The model under review builds one solid part; all positions refer to its coordinate system, in mm. Coordinates: 2 decimals unless noted, no trailing zeros. Order: outer loops, then holes, each group sorted by start corner. A loop starts at its lowest first (then second) coordinate and runs counter-clockwise, first axis right, second up. Notation, with made-up numbers: M 50.25,-11.75 L 57.25,-11.75 A12 ccw 57.25,2.25 Z; hole C 71.5,-5 d6. An arc over 180 degrees is marked long. Answer as CSV lines item,"result". Start each with the question number.
Q1. Wall thickness on L1, parallel to X at y = 230, z = -3; L2, parallel to X at y = 142.5, z = -1.6; L3, parallel to X at y = 96, z = -0.85: over which ranges is each line inside the solid? List them lowest first. Write a range as [from, to].
Q2. Consider section A-A on x = 41. Write out the cut boundary in (y, z), and give its area (3 significant figures).
Q3. Consider section B-B on y = 212.5. Write out the cut boundary in (x, z).
Autodesk Inventor part; units mm, degrees
ref_plane "YZ Plane" through (0, 0, 0) normal (1, 0, 0) x (0, 1, 0)
ref_plane "XZ Plane" through (0, 0, 0) normal (0, 1, 0) x (-1, 0, 0)
ref_plane "XY Plane" through (0, 0, 0) normal (0, 0, 1) x (1, 0, 0)
sketch "Sketch1" plane through (0, 0, 0) normal (0, 0, 1) x (1, 0, 0)
  line L0 (120, -66) -> (20, -66) construction
  line L1 (20, -66) -> (20, -26) construction
  line L2 (20, -26) -> (120, -26) construction
  line L3 (120, -26) -> (120, -66) construction
  line L4 (-275, -71) -> (125, -71) construction
  line L5 (125, -71) -> (125, 329) construction
  line L6 (125, 329) -> (-275, 329) construction
  line L7 (-275, 329) -> (-275, -71) construction
  line L8 (50, 104) -> (50, 154) construction
  line L9 (50, 154) -> (54, 154) construction
  line L10 (54, 154) -> (54, 104) construction
  line L11 (54, 104) -> (50, 104) construction
  line L12 (-50, 254) -> (-100, 254) construction
  line L13 (-100, 254) -> (-100, 258) construction
  line L14 (-100, 258) -> (-50, 258) construction
  line L15 (-50, 258) -> (-50, 254) construction
  line L16 (50, 258) -> (50, 254) construction
  line L17 (50, 254) -> (54, 254) construction
  line L18 (54, 254) -> (54, 204) construction
  line L19 (54, 204) -> (50, 204) construction
  line L20 (50, 204) -> (50, 254) construction
  line L21 (50, 254) -> (0, 254) construction
  line L22 (0, 254) -> (0, 258) construction
  line L23 (0, 258) -> (50, 258) construction
  line L24 (54, 4) -> (50, 4) construction
  line L25 (50, 4) -> (50, 0) construction
  line L26 (50, 0) -> (0, 0) construction
  line L27 (0, 0) -> (0, 4) construction
  line L28 (0, 4) -> (50, 4) construction
  line L29 (50, 4) -> (50, 54) construction
  line L30 (50, 54) -> (54, 54) construction
  line L31 (54, 54) -> (54, 4) construction
  line L32 (-100, 4) -> (-50, 4) construction
  line L33 (-50, 4) -> (-50, 0) construction
  line L34 (-50, 0) -> (-100, 0) construction
  line L35 (-100, 0) -> (-100, 4) construction
  line L36 (-204, 254) -> (-200, 254) construction
  line L37 (-200, 254) -> (-200, 258) construction
  line L38 (-200, 258) -> (-150, 258) construction
  line L39 (-150, 258) -> (-150, 254) construction
  line L40 (-150, 254) -> (-200, 254) construction
  line L41 (-200, 254) -> (-200, 204) construction
  line L42 (-200, 204) -> (-204, 204) construction
  line L43 (-204, 204) -> (-204, 254) construction
  line L44 (-200, 154) -> (-200, 104) construction
  line L45 (-200, 104) -> (-204, 104) construction
  line L46 (-204, 104) -> (-204, 154) construction
  line L47 (-204, 154) -> (-200, 154) construction
  line L48 (-200, 54) -> (-200, 4) construction
  line L49 (-200, 4) -> (-150, 4) construction
  line L50 (-150, 4) -> (-150, 0) construction
  line L51 (-150, 0) -> (-200, 0) construction
  line L52 (-200, 0) -> (-200, 4) construction
  line L53 (-200, 4) -> (-204, 4) construction
  line L54 (-204, 4) -> (-204, 54) construction
  line L55 (-204, 54) -> (-200, 54) construction
  line L56 (-275, -71) -> (125, -71) construction
  line L57 (125, -71) -> (125, 329) construction
  line L58 (125, 329) -> (-275, 329) construction
  line L59 (-275, 329) -> (-275, -71) construction
  line L60 (-275, -71) -> (125, 329) construction
  line L61 (75, 279) -> (-225, 279)
  line L62 (-225, 279) -> (-225, -21)
  line L63 (-225, -21) -> (75, -21)
  line L64 (75, -21) -> (75, 279)
  line L65 (75, 279) -> (-225, -21) construction
  line L66 (-225, 279) -> (75, -21) construction
  line L67 (-204, 4) -> (-200, 4)
  line L68 (-200, 4) -> (-200, 54)
  line L69 (-200, 54) -> (-204, 54)
  line L70 (-204, 54) -> (-204, 4)
  line L71 (-200, 104) -> (-204, 104)
  line L72 (-204, 104) -> (-204, 154)
  line L73 (-204, 154) -> (-200, 154)
  line L74 (-200, 154) -> (-200, 104)
  line L75 (-200, 204) -> (-204, 204)
  line L76 (-204, 204) -> (-204, 254)
  line L77 (-204, 254) -> (-200, 254)
  line L78 (-200, 254) -> (-200, 204)
  line L79 (-200, 254) -> (-150, 254)
  line L80 (-150, 254) -> (-150, 258)
  line L81 (-150, 258) -> (-200, 258)
  line L82 (-200, 258) -> (-200, 254)
  line L83 (-100, 254) -> (-50, 254)
  line L84 (-50, 254) -> (-50, 258)
  line L85 (-50, 258) -> (-100, 258)
  line L86 (-100, 258) -> (-100, 254)
  line L87 (0, 254) -> (50, 254)
  line L88 (50, 254) -> (50, 258)
  line L89 (50, 258) -> (0, 258)
  line L90 (0, 258) -> (0, 254)
  line L91 (50, 254) -> (54, 254)
  line L92 (54, 254) -> (54, 204)
  line L93 (54, 204) -> (50, 204)
  line L94 (50, 204) -> (50, 254)
  line L95 (54, 154) -> (50, 154)
  line L96 (50, 154) -> (50, 104)
  line L97 (50, 104) -> (54, 104)
  line L98 (54, 104) -> (54, 154)
  line L99 (54, 4) -> (50, 4)
  line L100 (50, 4) -> (50, 54)
  line L101 (50, 54) -> (54, 54)
  line L102 (54, 54) -> (54, 4)
  line L103 (50, 4) -> (0, 4)
  line L104 (0, 4) -> (0, 0)
  line L105 (0, 0) -> (50, 0)
  line L106 (50, 0) -> (50, 4)
  line L107 (-100, 0) -> (-50, 0)
  line L108 (-50, 0) -> (-50, 4)
  line L109 (-50, 4) -> (-100, 4)
  line L110 (-100, 4) -> (-100, 0)
  line L111 (-200, 0) -> (-150, 0)
  line L112 (-150, 0) -> (-150, 4)
  line L113 (-150, 4) -> (-200, 4)
  line L114 (-200, 4) -> (-200, 0)
  point P0 (-75, 129)
  dimension "d0" = 300
  dimension "d1" = 300
extrude "Extrusion1" add sketch "Sketch1" against normal blind 4
sketch "Sketch2" plane through (0, 0, 0) normal (0, 0, 1) x (1, 0, 0)
  line L0 (-175, 234) -> (-171, 234)
  line L1 (-171, 234) -> (-171, 184)
  line L2 (-171, 184) -> (-175, 184)
  line L3 (-175, 184) -> (-175, 234)
  line L4 (-175, 184) -> (-171, 184)
  line L5 (-171, 184) -> (-171, 134)
  line L6 (-171, 134) -> (-175, 134)
  line L7 (-175, 134) -> (-175, 184)
  line L8 (-175, 134) -> (-171, 134)
  line L9 (-171, 134) -> (-171, 84)
  line L10 (-171, 84) -> (-175, 84)
  line L11 (-175, 84) -> (-175, 134)
  line L12 (-200, 254) -> (-200, 204)
  line L13 (-150, 254) -> (-200, 254)
  line L14 (-175, 84) -> (-171, 84)
  line L15 (-171, 84) -> (-171, 34)
  line L16 (-171, 34) -> (-175, 34)
  line L17 (-175, 34) -> (-175, 84)
  line L18 (-175, 34) -> (-171, 34)
  line L19 (-171, 34) -> (-171, 24)
  line L20 (-171, 24) -> (-175, 24)
  line L21 (-175, 24) -> (-175, 34)
  line L22 (-200, 4) -> (-150, 4)
  line L23 (25, 184) -> (21, 184)
  line L24 (21, 184) -> (25, 184)
  line L25 (21, 234) -> (25, 234)
  line L26 (25, 234) -> (25, 184)
  line L27 (21, 184) -> (21, 234)
  line L28 (25, 184) -> (25, 134)
  line L29 (25, 134) -> (21, 134)
  line L30 (21, 134) -> (25, 134)
  line L31 (25, 134) -> (25, 84)
  line L32 (25, 84) -> (21, 84)
  line L33 (21, 84) -> (21, 134)
  line L34 (21, 134) -> (21, 184)
  line L35 (21, 84) -> (25, 84)
  line L36 (25, 84) -> (25, 34)
  line L37 (21, 34) -> (21, 84)
  line L38 (25, 34) -> (21, 34)
  line L39 (21, 34) -> (25, 34)
  line L40 (25, 34) -> (25, 24)
  line L41 (21, 24) -> (21, 34)
  line L42 (25, 24) -> (21, 24)
  point P0 (0, 0)
  point P1 (-173, 234)
  point P2 (-173, 24)
  point P3 (23, 234)
  point P4 (23, 24)
  dimension "d4" = 4
  dimension "d5" = 50
  dimension "d6" = 4
  dimension "d7" = 50
  dimension "d8" = 4
  dimension "d9" = 50
  dimension "d10" = 25
  dimension "d11" = 20
  dimension "d12" = 4
  dimension "d13" = 50
  dimension "d14" = 4
  dimension "d15" = 20
  dimension "d20" = 196
extrude "Extrusion2" cut sketch "Sketch2" against normal blind 10 contours L0 L1 L2 L3 | L6 L9 L10 L11 | L16 L19 L20 L21 | L23 L27 L25 L26 | L31 L32 L33 L29 | L40 L42 L41 L38
properties part number "Roof_V1"
Evaluation:
1,L1,"x = [-225, -204], [-200, -175], [-171, 21], [25, 50], [54, 75]"
1,L2,"x = [-225, -204], [-200, 50], [54, 75]"
1,L3,"x = [-225, -175], [-171, 21], [25, 75]"
2,outline,"M -21,-4 L 0,-4 L 0,0 L -21,0 Z; M 4,-4 L 254,-4 L 254,0 L 4,0 Z; M 258,-4 L 279,-4 L 279,0 L 258,0 Z"
2,area,"1,170 mm²"
3,outline,"M -225,-4 L -204,-4 L -204,0 L -225,0 Z; M -200,-4 L -175,-4 L -175,0 L -200,0 Z; M -171,-4 L 21,-4 L 21,0 L -171,0 Z; M 25,-4 L 50,-4 L 50,0 L 25,0 Z; M 54,-4 L 75,-4 L 75,0 L 54,0 Z"
